Input: part model. Units: mm. Frame: model coordinates. A direction names the side the tool comes from. Round coordinates to 2 decimals unless told otherwise and drop trailing zeros. Order: outer loops, then holes, each group sorted by start corner. A loop starts at its lowest first (then second) coordinate and runs counter-clockwise, first axis right, second up. Notation, with made-up numbers: (-30.5, 73) - (3.5, 73) arc R7 ccw to (3.5, 77) - close; hole circle Ø10 at (53.25, 13.5). An arc over 180 degrees is marked (long way). One line per item, written item: value. Start each with the question number.
from build123d import *

# Parameters (mm, degrees)
SKETCH1_W           = 914.4
SKETCH1_H           = 914.4
SKETCH1_R           = 3.175
BOSS_EXTRUDE1_DEPTH = 3.175
SKETCH4_W           = 914.4
SKETCH4_H           = 914.4
SKETCH4_W_2         = 908.05
SKETCH4_H_2         = 908.05
BOSS_EXTRUDE2_DEPTH = 50.8


with BuildPart() as part:
    # Sketch1 → Boss-Extrude1 (new body)
    with BuildSketch(Plane(origin=(0, 0, 0), x_dir=(1, 0, 0), z_dir=(0, 1, 0))):
        Rectangle(SKETCH1_W, SKETCH1_H)
        with Locations((-334.137, 406.4)):
            Circle(SKETCH1_R, mode=Mode.SUBTRACT)
        with Locations((-334.137, 279.4)):
            Circle(SKETCH1_R, mode=Mode.SUBTRACT)
        with Locations((-334.137, 152.4)):
            Circle(SKETCH1_R, mode=Mode.SUBTRACT)
        with Locations((-334.137, 25.4)):
            Circle(SKETCH1_R, mode=Mode.SUBTRACT)
        with Locations((-334.137, -101.6)):
            Circle(SKETCH1_R, mode=Mode.SUBTRACT)
        with Locations((334.137, -101.6)):
            Circle(SKETCH1_R, mode=Mode.SUBTRACT)
        with Locations((334.137, 25.4)):
            Circle(SKETCH1_R, mode=Mode.SUBTRACT)
        with Locations((334.137, 152.4)):
            Circle(SKETCH1_R, mode=Mode.SUBTRACT)
        with Locations((334.137, 279.4)):
            Circle(SKETCH1_R, mode=Mode.SUBTRACT)
        with Locations((334.137, 406.4)):
            Circle(SKETCH1_R, mode=Mode.SUBTRACT)
    extrude(amount=BOSS_EXTRUDE1_DEPTH)

    # Sketch4 → Boss-Extrude2 (add)
    with BuildSketch(Plane.XZ):
        Rectangle(SKETCH4_W, SKETCH4_H)
        Rectangle(SKETCH4_W_2, SKETCH4_H_2, mode=Mode.SUBTRACT)
    extrude(amount=BOSS_EXTRUDE2_DEPTH)


solid = part.part
1. Pull-direction query (Z, two-part tool) for faces 1 (the face through (-454.025, -25, -6)), 2 (the face through (-457.2, -23, -6)), 3 (the face through (-6, -23, -457.2)); classes: released by +Z, released by -Z, zero draft, split by the parting line, or undercut.
2. Set-up query: faces 4 (the face through (454.025, -25, -6)), 5 (the face through (-6, -23, 457.2)). Return all of +Z, -Z, +X, -X, +Y, -Y with unobstructed straight access to the full face (end or side cutting, diameter ignored); none if empty.
3. Section C-C (z = 397). Return the cut outline in (x, y) (3 decimals).
4. Line query: line 1 (X direction, y = 1, z = -406); line 2 (X direction, y = -43.5, z = -263) (3 decimals). Output: solid intervals per line, ascending. Write a range as from..to.
5. Section B-B (x = 243). Return the cut outline in (y, z) (3 decimals).
6. Section A-A (y = -12.5). Return the cut outline in (x, z) (3 decimals).
7. Pin query (flat end, axial travel): pin 1 (7.5 mm diameter, centred on x = 334.137, z = -152.4, fed in from -Y); pin 2 (8.5 mm diameter, centred on x = 334.137, z = -279.4, fed in from +Y) (3 decimals). Return the tip coordinate at first contact, or that it passes through.
Solved:
1. face 1: undercut
1. face 2: zero draft
1. face 3: released by -Z
2. face 4: -Y
2. face 5: +Z, +X, -X, +Y, -Y
3. outline: (-457.2, -50.8) - (-454.025, -50.8) - (-454.025, 0) - (454.025, 0) - (454.025, -50.8) - (457.2, -50.8) - (457.2, 3.175) - (-457.2, 3.175) - close
4. line 1: x = -457.2..-337.29, -330.99..330.99, 337.29..457.2
4. line 2: x = -457.2..-454.025, 454.025..457.2
5. outline: (-50.8, -457.2) - (3.175, -457.2) - (3.175, 457.2) - (-50.8, 457.2) - (-50.8, 454.025) - (0, 454.025) - (0, -454.025) - (-50.8, -454.025) - close
6. outline: (-457.2, -457.2) - (457.2, -457.2) - (457.2, 457.2) - (-457.2, 457.2) - close; hole (-454.025, -454.025) - (454.025, -454.025) - (454.025, 454.025) - (-454.025, 454.025) - close
7. pin 1: stops at y = 0
7. pin 2: stops at y = 3.175
